Work out the finished part from the listing and answer in its coordinate system (mm). Face numbers are marked on the shaded views. A direction names the side the tool comes from. Coordinates: 2 decimals unless noted, no trailing zeros. Order: outer loops, then holes, each group sorted by start corner. A loop starts at its lowest first (then second) coordinate and runs counter-clockwise, first axis right, second up.
1. A flat-ended cylindrical pin translates along its axis: pin 1 Ø0.6 at (x, z) = (12.5, -2) entering from +Y (3 decimals). Find the tip coordinate at first contact, or state that the pin passes through.
2. Find the intervals of material crossed by probe 1 along X at (y, z) = (-0.7, 0); probe 2 along Z at (x, y) = (0, -0.65); probe 3 along Y at (x, z) = (11, -0.25) (3 decimals), in increasing order.
3. The part is cut by section B-B, the plane y = -0.65. Give the vertices of the cut face in (x, z).
4. A tool of negligible diameter and unlimited length cuts with its end or side. For the marked faces 4 and 5, from which of +Z, -Z, +X, -X, +Y, -Y can it reach the whole face along a straight path? Write none if from no direction.
5. Determine the mould class of the marked faces 1, 2 and 3 for opening direction X: +X half, -X half, draft (parallel to the pull), parting line (faces both ways), or undercut.
6. The part is cut by section A-A, the plane x = 0. Give the vertices of the cut face in (y, z) (3 decimals), then the cut area to 4 significant figures.
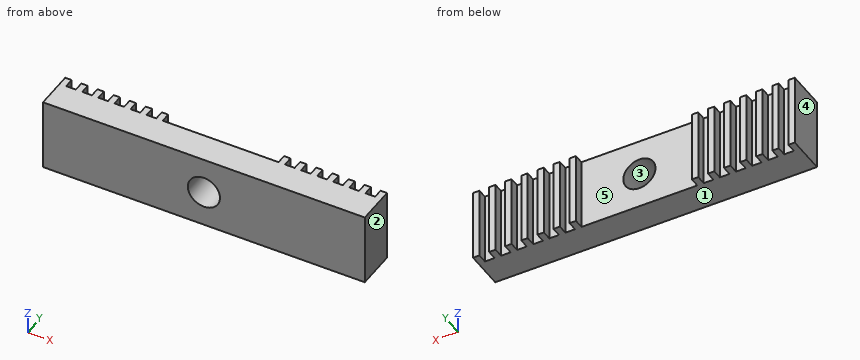
Autodesk Inventor part; units mm, degrees
ref_plane "YZ Plane" through (0, 0, 0) normal (1, 0, 0) x (0, 1, 0)
ref_plane "XZ Plane" through (0, 0, 0) normal (0, 1, 0) x (-1, 0, 0)
ref_plane "XY Plane" through (0, 0, 0) normal (0, 0, 1) x (1, 0, 0)
sketch "Sketch1" plane through (0, 0, 0) normal (0, 0, 1) x (1, 0, 0)
  line L0 (-20, 2.425) -> (-19.2, 2.425)
  line L1 (0, -2.425) -> (-20, -2.425)
  line L2 (-20, -2.425) -> (-20, 2.425)
  line L3 (-18, 2.425) -> (-18, 1.225)
  line L4 (-18, 1.225) -> (-19.2, 1.225)
  line L5 (-19.2, 1.225) -> (-19.2, 2.425)
  line L6 (-16, 2.425) -> (-16, 1.225)
  line L7 (-16, 1.225) -> (-17.2, 1.225)
  line L8 (-17.2, 1.225) -> (-17.2, 2.425)
  line L9 (-14, 2.425) -> (-14, 1.225)
  line L10 (-14, 1.225) -> (-15.2, 1.225)
  line L11 (-15.2, 1.225) -> (-15.2, 2.425)
  line L12 (-12, 2.425) -> (-12, 1.225)
  line L13 (-12, 1.225) -> (-13.2, 1.225)
  line L14 (-13.2, 1.225) -> (-13.2, 2.425)
  line L15 (-10, 2.425) -> (-10, 1.225)
  line L16 (-10, 1.225) -> (-11.2, 1.225)
  line L17 (-11.2, 1.225) -> (-11.2, 2.425)
  line L18 (-20, 1.225) -> (0, 1.225) construction
  line L19 (0, 0) -> (-20, 0) construction
  line L20 (-8, 2.425) -> (-8, 1.225)
  line L21 (-8, 1.225) -> (-9.2, 1.225)
  line L22 (-9.2, 1.225) -> (-9.2, 2.425)
  line L23 (0, 1.225) -> (-7.2, 1.225)
  line L24 (-7.2, 1.225) -> (-7.2, 2.425)
  line L25 (-18, 2.425) -> (-17.2, 2.425)
  line L26 (-16, 2.425) -> (-15.2, 2.425)
  line L27 (-14, 2.425) -> (-13.2, 2.425)
  line L28 (-12, 2.425) -> (-11.2, 2.425)
  line L29 (-10, 2.425) -> (-9.2, 2.425)
  line L30 (-8, 2.425) -> (-7.2, 2.425)
  line L31 (0, 1.225) -> (0, -2.425) construction
  line L32 (20, 2.425) -> (19.2, 2.425)
  line L33 (0, -2.425) -> (20, -2.425)
  line L34 (20, -2.425) -> (20, 2.425)
  line L35 (18, 2.425) -> (18, 1.225)
  line L36 (18, 1.225) -> (19.2, 1.225)
  line L37 (19.2, 1.225) -> (19.2, 2.425)
  line L38 (16, 2.425) -> (16, 1.225)
  line L39 (16, 1.225) -> (17.2, 1.225)
  line L40 (17.2, 1.225) -> (17.2, 2.425)
  line L41 (14, 2.425) -> (14, 1.225)
  line L42 (14, 1.225) -> (15.2, 1.225)
  line L43 (15.2, 1.225) -> (15.2, 2.425)
  line L44 (12, 2.425) -> (12, 1.225)
  line L45 (12, 1.225) -> (13.2, 1.225)
  line L46 (13.2, 1.225) -> (13.2, 2.425)
  line L47 (10, 2.425) -> (10, 1.225)
  line L48 (10, 1.225) -> (11.2, 1.225)
  line L49 (11.2, 1.225) -> (11.2, 2.425)
  line L50 (20, 1.225) -> (0, 1.225) construction
  line L51 (0, 0) -> (20, 0) construction
  line L52 (8, 2.425) -> (8, 1.225)
  line L53 (8, 1.225) -> (9.2, 1.225)
  line L54 (9.2, 1.225) -> (9.2, 2.425)
  line L55 (0, 1.225) -> (7.2, 1.225)
  line L56 (7.2, 1.225) -> (7.2, 2.425)
  line L57 (18, 2.425) -> (17.2, 2.425)
  line L58 (16, 2.425) -> (15.2, 2.425)
  line L59 (14, 2.425) -> (13.2, 2.425)
  line L60 (12, 2.425) -> (11.2, 2.425)
  line L61 (10, 2.425) -> (9.2, 2.425)
  line L62 (8, 2.425) -> (7.2, 2.425)
  dimension "d0" = 4.85
  dimension "d3" = 1.2
  dimension "d4" = 0.8
  dimension "d5" = 1.2
  dimension "d6" = 0.8
  dimension "d7" = 1.2
  dimension "d8" = 0.8
  dimension "d9" = 1.2
  dimension "d10" = 0.8
  dimension "d13" = 0.8
  dimension "d14" = 1.2
  dimension "d15" = 0.8
  dimension "d16" = 1.2
  dimension "d17" = 0.8
  dimension "d18" = 40
  dimension "d19" = 3.65
extrude "Extrusion1" add sketch "Sketch1" along normal mid plane 9
sketch "Sketch2" plane through (0, 0, 0) normal (0, 1, 0) x (-1, 0, 0)
  circle A0 centre (0, 0) radius 2.2937
  circle A1 centre (0, 0) radius 2
  dimension "d22" = 4
extrude "Extrusion2" cut sketch "Sketch2" along normal through all both and the other way through all contours A1
equation "\"d5\" = d3"
equation "\"d7\" = d3"
equation "\"d8\" = d4"
equation "\"d9\" = d3"
equation "\"d10\" = d4"
equation "\"d13\" = d4"
equation "\"d14\" = d3"
equation "\"d15\" = d4"
equation "\"d16\" = d3"
equation "\"d17\" = d4"
properties part number "fixador-correia" material "Steel, Cast"
Geometry says:
1. pin 1: stops at y = 1.225
2. probe 1: x = -20 to -2, 2 to 20
2. probe 2: z = -4.5 to -2, 2 to 4.5
2. probe 3: y = -2.425 to 1.225
3. outline: (-20, -4.5) - (20, -4.5) - (20, 4.5) - (-20, 4.5) - close; hole circle Ø4 at (0, 0)
4. face 4: +Z, -Z, -X, +Y, -Y
4. face 5: +Z, -Z, +Y
5. face 1: draft
5. face 2: +X half
5. face 3: undercut
6. outline: (-2.425, -4.5) - (1.225, -4.5) - (1.225, -2) - (-2.425, -2) - close; (-2.425, 2) - (1.225, 2) - (1.225, 4.5) - (-2.425, 4.5) - close
6. area: 18.25 mm2
